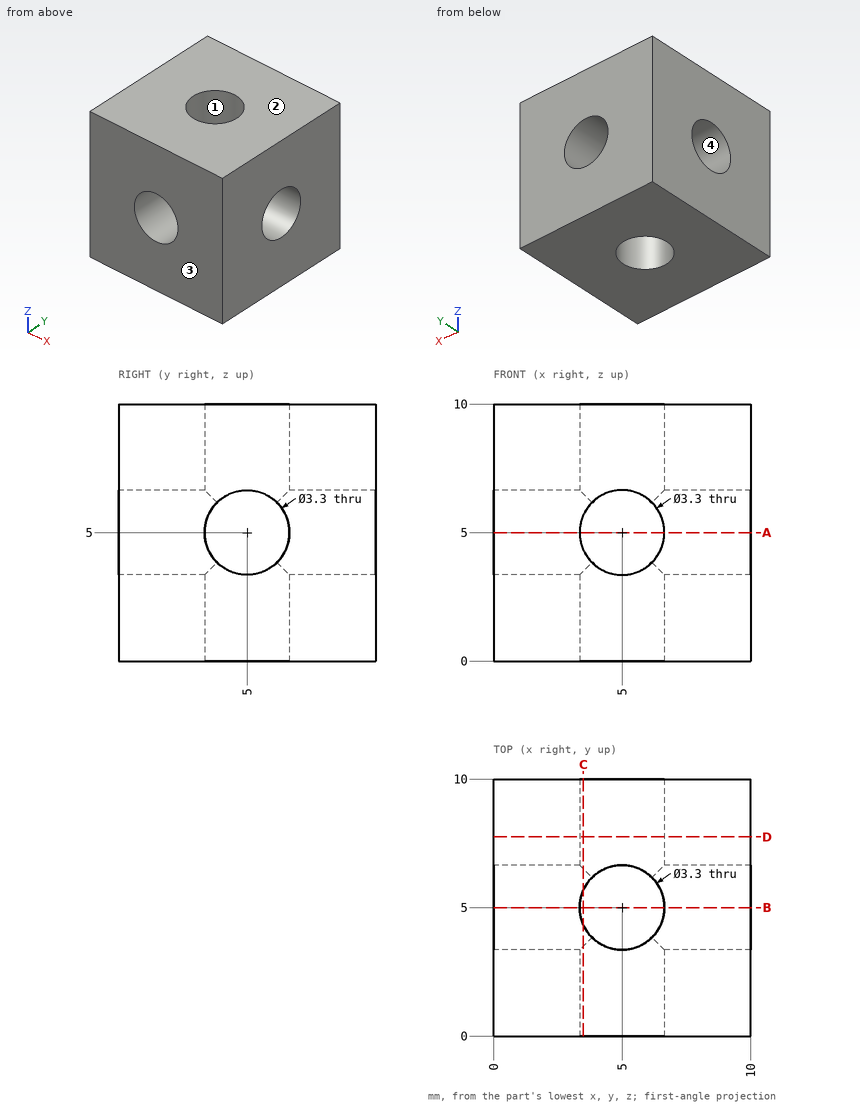
The drawing under review shows one solid part. Ordinate dimensions are in mm from its lowest x, y, z. Give positions to 0.01 mm unless a question says otherwise; leave off trailing zeros. Order: outer loops, then holes, each group sorted by start corner. A loop starts at its lowest first (then second) coordinate and runs counter-clockwise, first axis right, second up. Notation, with made-up numbers: (-34, 39) -> (12, 39) arc R19 ccw to (12, 47) -> close; hole circle Ø1 at (32.25, -22.5). An arc over 180 degrees is marked (long way). Write item = value, one per line. Start each with the question number.
(1) To check wall thickness, follow line 1 along Y through (x, z) = (5, 7.5). State the ranges of the line that lie inside material, in increasing order.
(2) We need section C-C on x = 3.5. Write out the cut boundary in (y, z).
(3) Mouldability with a two-part tool opening along Y and no side actions: class the marked faces 1, 2, 3 and 4 as +Y half, -Y half, draft (parallel to the pull), parting line (faces both ways), or undercut.
(4) We need section A-A on z = 5. Write out the cut boundary in (x, y).
(5) We need section D-D on y = 7.75. Write out the cut boundary in (x, z).
(6) For pin 1 (3 mm diameter, centred on y = 5, z = 5, fed in from +X), flat-tipped, find the tip position at first contact; note if it passes through.
Numbers:
q1.line_1 = 0 to 3.35, 6.65 to 10
q2.outline = (0, 0) -> (4.31, 0) -> (4.31, 3.5) arc R1.65 cw to (3.5, 4.31) -> (0, 4.31) -> close; (0, 5.69) -> (3.5, 5.69) arc R1.65 cw to (4.31, 6.5) -> (4.31, 10) -> (0, 10) -> close; (5.69, 0) -> (10, 0) -> (10, 4.31) -> (6.5, 4.31) arc R1.65 cw to (5.69, 3.5) -> close; (5.69, 6.5) arc R1.65 cw to (6.5, 5.69) -> (10, 5.69) -> (10, 10) -> (5.69, 10) -> close
q3.face_1 = undercut
q3.face_2 = draft
q3.face_3 = -Y half
q3.face_4 = undercut
q4.outline = (0, 0) -> (3.35, 0) -> (3.35, 3.35) -> (0, 3.35) -> close; (0, 6.65) -> (3.35, 6.65) -> (3.35, 10) -> (0, 10) -> close; (6.65, 0) -> (10, 0) -> (10, 3.35) -> (6.65, 3.35) -> close; (6.65, 6.65) -> (10, 6.65) -> (10, 10) -> (6.65, 10) -> close
q5.outline = (0, 0) -> (10, 0) -> (10, 10) -> (0, 10) -> close; hole circle Ø3.3 at (5, 5)
q6.pin_1 = through
